```python
from build123d import *

# Parameters (mm, degrees)
SKETCH1_R           = 8
BOSS_EXTRUDE1_DEPTH = 3
CUT_EXTRUDE1_DEPTH  = 133.578278764
CUT_EXTRUDE8_DEPTH  = 10
FILLET2_R           = 5
FILLET3_R           = 5
FILLET4_R           = 5
SKETCH6_R           = 9.723108926
SKETCH6_R_2         = 1
BOSS_EXTRUDE2_DEPTH = 3
SKETCH10_R          = 1
CUT_EXTRUDE9_DEPTH  = 10


with BuildPart() as part:
    # Sketch1 → Boss-Extrude1 (new body)
    with BuildSketch(Plane.XY):
        with BuildLine():
            Line((0, -12), (-120, -12))
            ThreePointArc((-120, -12), (-132, 0), (-120, 12))
            Line((-120, 12), (0, 12))
            ThreePointArc((0, 12), (12, 0), (0, -12))
        make_face()
        with Locations((-120, 0)):
            Circle(SKETCH1_R, mode=Mode.SUBTRACT)
        with Locations(Location((0, 0, 0), (0, 0, 180))):
            Circle(SKETCH1_R, mode=Mode.SUBTRACT)
    extrude(amount=BOSS_EXTRUDE1_DEPTH)

    # Sketch2 → Cut-Extrude1 (cut, through all)
    with BuildSketch(Plane.XY.offset(3)):
        with BuildLine():
            Line((-17.036725037, 6), (-20.036725037, 6))
            ThreePointArc((-20.036725037, 6), (-18.824439071, 9.116514898), (-17.130976336, 12))
            Line((-17.130976336, 12), (-13.5, 12))
            ThreePointArc((-13.5, 12), (-15.560298648, 9.172082969), (-17.036725037, 6))
        make_face()
        with BuildLine():
            Line((-102.963274963, 6), (-99.963274963, 6))
            ThreePointArc((-99.963274963, 6), (-101.175560929, 9.116514898), (-102.869023664, 12))
            Line((-102.869023664, 12), (-106.5, 12))
            ThreePointArc((-106.5, 12), (-104.439701352, 9.172082969), (-102.963274963, 6))
        make_face()
    extrude(amount=-CUT_EXTRUDE1_DEPTH, mode=Mode.SUBTRACT)

    # Sketch5 → Cut-Extrude8 (cut)
    with BuildSketch(Plane.XY.offset(3)):
        with BuildLine():
            Line((-1.731193523, -11.858337769), (-1.731193523, -12))
            Line((-1.731193523, -12), (-22.731193523, -12))
            Line((-22.731193523, -12), (-22.731193523, -2.344249067))
            Line((-22.731193523, -2.344249067), (-22.731193523, -1.572214532))
            Line((-22.731193523, -1.572214532), (-11.880460729, -1.572214532))
            ThreePointArc((-11.880460729, -1.572214532), (-8.530554828, -8.417056492), (-1.731193523, -11.858337769))
        make_face()
    extrude(amount=-CUT_EXTRUDE8_DEPTH, mode=Mode.SUBTRACT)

    # Fillet2
    fillet2_edges = [part.edges().sort_by_distance(p)[0] for p in [
        (-22.731193523, -1.572214532, 1.5),
    ]]
    fillet(fillet2_edges, radius=FILLET2_R)

    # Fillet3
    fillet3_edges = [part.edges().sort_by_distance(p)[0] for p in [
        (-11.880460729, -1.572214532, 1.5),
    ]]
    fillet(fillet3_edges, radius=FILLET3_R)

    # Fillet4
    fillet4_edges = [part.edges().sort_by_distance(p)[0] for p in [
        (-22.731193523, -12, 1.5),
    ]]
    fillet(fillet4_edges, radius=FILLET4_R)

    # Sketch6 → Boss-Extrude2 (add)
    with BuildSketch(Plane.XY.offset(3)):
        Circle(SKETCH6_R)
        Circle(SKETCH6_R_2, mode=Mode.SUBTRACT)
    extrude(amount=-BOSS_EXTRUDE2_DEPTH)

    # Sketch10 → Cut-Extrude9 (cut)
    with BuildSketch(Plane(origin=(0, 0, 0), x_dir=(-1, 0, 0), z_dir=(0, 0, -1))):
        with Locations((0, 10.5)):
            Circle(SKETCH10_R)
        with Locations((0, 7.5)):
            Circle(SKETCH10_R)
        with Locations((0, -7.5)):
            Circle(SKETCH10_R)
        with Locations((0, -10.5)):
            Circle(SKETCH10_R)
    extrude(amount=-CUT_EXTRUDE9_DEPTH, mode=Mode.SUBTRACT)


solid = part.part
```
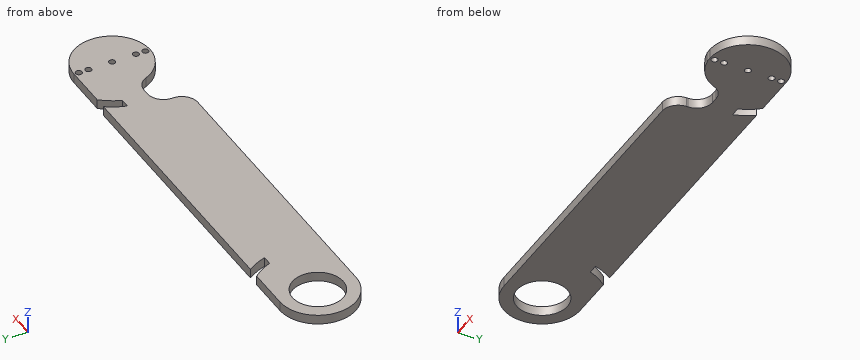
Here's how the part is built. I have some questions about the finished solid (model axes, mm). Give positions to 0.01 mm unless a question says otherwise; leave off trailing zeros. Order: outer loops, then holes, each group sorted by start corner. A loop starts at its lowest first (then second) coordinate and runs counter-clockwise, first axis right, second up. Notation, with made-up numbers: (78, 76) - (97, 76) arc R13 ccw to (97, 98) - close; hole circle Ø5 at (18, -32.75). An arc over 180 degrees is marked (long way). Answer as a JSON object with one key per item and string values. Group by question number.
Item 1: Please list where these lines run through material, in increasing order: probe 1 along Y at (x, z) = (0, 1.8); probe 2 along X at (y, z) = (-3.5, 1); probe 3 along X at (y, z) = (1.5, 0.25).
Item 2: If we section it at A-A on z = 1.3: Please give me the cut outline in (x, y).
Item 3: For P1, Ø1.7, axis at x = -17, z = 1, coming from the -Y side; P2, Ø0.5, axis at y = -7, z = 1.5, coming from the +X side; P3, Ø13, axis at x = -120, y = 0, coming from the -Z side; P4, Ø1, axis at y = -4, z = 1, coming from the +X side, each with a flat end and sliding along its axis, tell me the tip position at first contact or that it passes through.
Result set:
{
 "1": {"probe 1": "-12 to -11.5, -9.5 to -8.5, -6.5 to -1, 1 to 6.5, 8.5 to 9.5, 11.5 to 12", "probe 2": "-131.48 to -127.19, -112.81 to -21.68, -11.72 to 11.48", "probe 3": "-131.91 to -127.86, -112.14 to 11.91"},
 "2": {"outline": "(-120, -12) - (-27.73, -12) arc R5 ccw to (-22.73, -7) - (-22.73, -6.57) arc R5 cw to (-17.73, -1.57) - (-15.66, -1.57) arc R5 cw to (-11.05, -4.64) arc R11.98 ccw to (-1.73, -11.86) - (-1.73, -12) - (0, -12) arc R12 ccw to (0, 12) - (-13.5, 12) arc R18.06 ccw to (-17.04, 6) - (-20.04, 6) arc R20.92 cw to (-17.13, 12) - (-102.87, 12) arc R20.92 cw to (-99.96, 6) - (-102.96, 6) arc R18.06 ccw to (-106.5, 12) - (-120, 12) arc R12 ccw to start; hole circle Ø16 at (-120, 0); hole circle Ø2 at (0, -10.5); hole circle Ø2 at (0, -7.5); hole circle Ø2 at (0, 0); hole circle Ø2 at (0, 7.5); hole circle Ø2 at (0, 10.5)"},
 "3": {"P1": "y = -1.57", "P2": "x = 9.92", "P3": "through", "P4": "x = 11.48"}
}
